from build123d import *

# Parameters (mm, degrees)
SKETCH1_R           = 2.5
BOSS_EXTRUDE1_DEPTH = 2
CUT_EXTRUDE1_DEPTH  = 10


with BuildPart() as part:
    # Sketch1 → Boss-Extrude1 (new body)
    with BuildSketch(Plane.XY.offset(92)):
        Polygon((26.130057398, -8.597379557), (26.130057398, -23.597379557), (83.470700498, -63.747730101), (402.6593569, -63.747730101), (460, -23.597379557), (460, -8.597379557), align=None)
        with Locations((173.065028699, -41.747730101)):
            Circle(SKETCH1_R, mode=Mode.SUBTRACT)
        with Locations((313.065028699, -41.747730101)):
            Circle(SKETCH1_R, mode=Mode.SUBTRACT)
    extrude(amount=BOSS_EXTRUDE1_DEPTH)

    # Sketch2 → Cut-Extrude1 (cut)
    with BuildSketch(Plane(origin=(0, 0, 92), x_dir=(-1, 0, 0), z_dir=(0, 0, -1))):
        Polygon((-381.8278919, -8.597379557), (-360.405671799, -23.597379557), (-360.405671799, -8.597379557), align=None)
        Polygon((-303.065028699, -63.747730101), (-360.405671799, -23.597379557), (-381.8278919, -8.597379557), (-460, -8.597379557), (-460, -23.597379557), (-402.6593569, -63.747730101), align=None)
        Polygon((-125.724385599, -8.597379557), (-125.724385599, -23.597379557), (-104.302165498, -8.597379557), align=None)
        Polygon((-104.302165498, -8.597379557), (-125.724385599, -23.597379557), (-183.065028699, -63.747730101), (-83.470700498, -63.747730101), (-26.130057398, -23.597379557), (-26.130057398, -8.597379557), align=None)
    extrude(amount=-CUT_EXTRUDE1_DEPTH, mode=Mode.SUBTRACT)


solid = part.part
The model under review builds one solid part; all positions refer to its coordinate system, in mm. Round coordinates to 2 decimals unless told otherwise and drop trailing zeros. Loops run counter-clockwise (first coordinate to the right, second up) from the corner with the lowest first, then second, coordinate; pieces in that order, holes last. Notation, with made-up numbers: (68, 40) -> (115, 40) arc R20 ccw to (115, 67) -> close; hole circle Ø3 at (49, 79). An arc over 180 degrees is marked (long way). One line per question, with ' | ' between items. Start each with the question number.
Item 1: Draft analysis for pull direction X (two halves, no side actions). For faces 1 (the face through (241, -30, 94)), 2 (the face through (174.41, -39.64, 92.99)), 3 (the face through (331.334, -43.954, 92.986)), state which applies: +X half, -X half, draft (parallel to the pull), parting line (faces both ways), or undercut.
Item 2: Add section A-A, the plane z = 93.6. Write out the cut boundary in (x, y).
Item 3: Add section B-B, the plane y = -48. Write out the cut boundary in (x, z), then the cut area to 3 significant figures.
Item 4: For pin 1 (3 mm diameter, centred on x = 173.07, y = -41.75, fed in from +Z), flat-tipped, find the tip position at first contact; note if it passes through.
Item 5: Add section C-C, the plane x = 322. Write out the cut boundary in (y, z).
Item 6: Wall thickness on line 1 along X through (y, z) = (-43.5, 92.85); line 2 along X through (y, z) = (-44, 92.85); line 3 along Y through (x, z) = (329, 93.45): over which ranges is each line inside the solid? List them lowest first. Write a range as [from, to].
Return value:
1) face 1: draft | face 2: undercut | face 3: +X half
2) outline: (125.72, -23.6) -> (183.07, -63.75) -> (303.07, -63.75) -> (360.41, -23.6) -> (360.41, -8.6) -> (125.72, -8.6) -> close; hole circle Ø5 at (173.07, -41.75); hole circle Ø5 at (313.07, -41.75)
3) outline: (160.57, 92) -> (325.56, 92) -> (325.56, 94) -> (160.57, 94) -> close | area: 330 mm2
4) pin 1: passes through
5) outline: (-50.49, 92) -> (-8.6, 92) -> (-8.6, 94) -> (-50.49, 94) -> close
6) line 1: x = [154.15, 171.28], [174.85, 311.28], [314.85, 331.98] | line 2: x = [154.86, 171.98], [174.15, 311.98], [314.15, 331.27] | line 3: y = [-45.59, -8.6]
